Here's how the part is built. I have some questions about the finished solid (model axes, mm). A direction names the side the tool comes from. Round coordinates to 2 decimals unless told otherwise and drop trailing zeros. Write each loop counter-clockwise with the first axis right and the second up, starting at its lowest first coordinate (ties: lowest second). Pieces come first, ordered by that corner, then holes. Notation, with made-up numbers: M 61,-28.75 L 78,-28.75 A14 ccw 78,-2.75 Z; hole C 29,9.25 d2. An arc over 180 degrees is marked long. Write item = value, one per line. Start each with the question number.
(1) On a 3-axis mill with a long thin cutter (end or side, diameter ignored), from which of +Z, -Z, +X, -X, +Y, -Y can I reach the whole of each face in a straight line? I mean faces 1 (the flat face through (0, 25, 0)), 2 (the flat face through (-21.5, 14, -2)), 3 (the flat face through (18, 33, -21.75)), 4 (the cylindrical face through (-14.93, 4.52, 10.5)). Say none if no direction works.
(2) I want a section at C-C (y = 48). List the corners of the cut face in (x, z) for me, and give its area (3 significant figures).
(3) Will these pins go through, and if not, where does the flat tip stop? pin 1 Ø3 at (x, y) = (-16, 33.5) entering from +Z; pin 2 Ø6 at (x, z) = (3.5, -11.5) entering from +Y; pin 3 Ø1.4 at (x, z) = (-1.5, -29) entering from +Y; pin 4 Ø8 at (x, z) = (-12.5, -7) entering from -Y.
(4) I want a section at B-B (x = 0). List the corners of the cut face in (y, z) for me, and give its area (3 significant figures).
(5) I need wall thicknesses on line 1 along Z through (x, y) = (-15, 4.85); line 2 along Y through (x, z) = (-6.5, 17.5); line 3 along Z through (x, y) = (-11, 15). Which ranges of each line are inside material? Lowest first, please.
(6) If we mould it in two halves opening along Y, with no side actions, what happens to faces 5 (the conical face through (-15.159, 6.745, 12.207)), 6 (the flat face through (17.24, 1.48, 10.68)), 7 (the cylindrical face through (-15.268, 29.367, -20.614))? For each: released by +Y, released by -Y, zero draft, split by the parting line, or undercut.
(7) I want a section at D-D (y = 11.5). List the corners of the cut face in (x, z) for me.
(8) I want a section at A-A (z = 17.5). List the corners of the cut face in (x, y) for me, and give its area (3 significant figures).
```python
from build123d import *

# Parameters (mm, degrees)
SKETCH9_W                 = 43
SKETCH9_H                 = 27
BOSS_EXTRUDE1_DEPTH       = 32.5
CUT_EXTRUDE1_DEPTH        = 61.284741021
CUT_EXTRUDE1_DEPTH_BACK   = 61.284741021
SKETCH10_R                = 6
CUT_EXTRUDE2_DEPTH        = 3
CUT_EXTRUDE4_DEPTH        = 61.284741021
CUT_EXTRUDE4_DEPTH_BACK   = 61.284741021
SKETCH14_W                = 30
SKETCH14_H                = 2
SKETCH15_W                = 43
SKETCH15_H                = 6
BOSS_EXTRUDE2_DEPTH       = 43
F_3_0MM_DOWEL_HOLE1_D     = 3
F_3_0MM_DOWEL_HOLE1_DEPTH = 6
F_3_0MM_DOWEL_HOLE1_TIP   = 0.901290929
FILLET2_R                 = 10
SKETCH20_R                = 11
CUT_EXTRUDE5_DEPTH        = 2
CUT_EXTRUDE6_DEPTH        = 95.827804467
CUT_EXTRUDE6_DEPTH_BACK   = 95.827804467
SKETCH21_R                = 5
SKETCH21_R_2              = 1.5
SKETCH23_R                = 3
CUT_EXTRUDE7_DEPTH        = 6


with BuildPart() as part:
    # Sketch9 → Boss-Extrude1 (new, symmetric)
    with BuildSketch(Plane.XY):
        with Locations((0, 13.5)):
            Rectangle(SKETCH9_W, SKETCH9_H)
    extrude(amount=BOSS_EXTRUDE1_DEPTH, both=True)

    # Sketch10 → Cut-Extrude1 (cut, two sides: drawn at the far end of the back side and taken through both)
    with BuildSketch(Plane(origin=(21.5, 0, 0), x_dir=(0, 0, -1), z_dir=(1, 0, 0)).offset(-CUT_EXTRUDE1_DEPTH_BACK)):
        with Locations((-17.5, 15)):
            Circle(SKETCH10_R)
        with Locations(Location((17.5, 15, 0), (0, 0, 270))):
            Circle(SKETCH10_R)
    extrude(amount=CUT_EXTRUDE1_DEPTH + CUT_EXTRUDE1_DEPTH_BACK, mode=Mode.SUBTRACT)

    # Sketch11 → Cut-Extrude2 (cut)
    with BuildSketch(Plane.XZ):
        Polygon((12, -12), (13.5, -9.401923789), (16.5, -9.401923789), (18, -12), (16.5, -14.598076211), (13.5, -14.598076211), align=None)
        Polygon((13.5, 9.401923789), (16.5, 9.401923789), (18, 12), (16.5, 14.598076211), (13.5, 14.598076211), (12, 12), align=None)
        Polygon((-13.5, -9.401923789), (-16.5, -9.401923789), (-18, -12), (-16.5, -14.598076211), (-13.5, -14.598076211), (-12, -12), align=None)
        Polygon((-12, 12), (-13.5, 9.401923789), (-16.5, 9.401923789), (-18, 12), (-16.5, 14.598076211), (-13.5, 14.598076211), align=None)
    extrude(amount=-CUT_EXTRUDE2_DEPTH, mode=Mode.SUBTRACT)

    # Sketch14 → Cut-Extrude4 (cut, two sides: drawn at the far end of the back side and taken through both)
    with BuildSketch(Plane(origin=(21.5, 0, 0), x_dir=(0, 0, -1), z_dir=(1, 0, 0)).offset(-CUT_EXTRUDE4_DEPTH_BACK)):
        with Locations((0, 26)):
            Rectangle(SKETCH14_W, SKETCH14_H)
    extrude(amount=CUT_EXTRUDE4_DEPTH + CUT_EXTRUDE4_DEPTH_BACK, mode=Mode.SUBTRACT)

    # Sketch15 → Boss-Extrude2 (add)
    with BuildSketch(Plane(origin=(0, 27, 0), x_dir=(1, 0, 0), z_dir=(0, 1, 0))):
        with Locations((0, 24.75)):
            Rectangle(SKETCH15_W, SKETCH15_H)
    extrude(amount=BOSS_EXTRUDE2_DEPTH)

    # Ø3.0mm Dowel Hole1
    with Locations(Plane(origin=(15, 0, 12), x_dir=(0, 0, -1), z_dir=(0, -1, 0))):
        with Locations((0, 0), (0, -30), (24, -30), (24, 0)):
            Hole(F_3_0MM_DOWEL_HOLE1_D / 2, depth=F_3_0MM_DOWEL_HOLE1_DEPTH)
            with Locations((0, 0, -(F_3_0MM_DOWEL_HOLE1_DEPTH + F_3_0MM_DOWEL_HOLE1_TIP / 2))):  # 118° drill point
                Cone(0, F_3_0MM_DOWEL_HOLE1_D / 2, F_3_0MM_DOWEL_HOLE1_TIP, mode=Mode.SUBTRACT)

    # Fillet2
    # the kernel refuses this fillet: 10 mm, written as the material it adds along each edge
    with BuildSketch(Plane(origin=(21.5, 27, -21.75), x_dir=(0, 0, 1), z_dir=(-1, 0, 0))) as fillet2_piece_1:
        with BuildLine():
            CenterArc((10, 9.45714016), FILLET2_R, 180, 71.034425011)
            Line((0, 9.45714016), (-0.2, 9.45714016))
            Line((-0.2, 9.45714016), (-0.2, 0))
            Line((-0.2, 0), (0, -0.2))
            ThreePointArc((0, -0.2), (3.375, -0.2), (6.685, -0.189142803))
            Line((6.685, -0.189142803), (6.75, 0))
        make_face()
    extrude(amount=43)

    # Sketch20 → Cut-Extrude5 (cut)
    with BuildSketch(Plane(origin=(0, 0, -27.75), x_dir=(-1, 0, 0), z_dir=(0, 0, -1))):
        with Locations((0, 48)):
            Circle(SKETCH20_R)
    extrude(amount=-CUT_EXTRUDE5_DEPTH, mode=Mode.SUBTRACT)

    # Sketch21 → Cut-Extrude6 (cut, two sides: drawn at the far end of the back side and taken through both)
    with BuildSketch(Plane(origin=(0, 0, -27.75), x_dir=(-1, 0, 0), z_dir=(0, 0, -1)).offset(-CUT_EXTRUDE6_DEPTH_BACK)):
        with Locations((0, 48)):
            Circle(SKETCH21_R)
        with Locations((-16.341750707, 64.341750707)):
            Circle(SKETCH21_R_2)
        with Locations((15.658249293, 64.341750707)):
            Circle(SKETCH21_R_2)
        with Locations((15.658249293, 32.341750707)):
            Circle(SKETCH21_R_2)
        with Locations((-16.341750707, 32.341750707)):
            Circle(SKETCH21_R_2)
    extrude(amount=CUT_EXTRUDE6_DEPTH + CUT_EXTRUDE6_DEPTH_BACK, mode=Mode.SUBTRACT)

    # Sketch23 → Cut-Extrude7 (cut)
    with BuildSketch(Plane.XY.offset(-21.75)):
        with Locations(Location((-15.658249293, 32.341750707, 0), (0, 0, 180))):
            Circle(SKETCH23_R)
        with Locations(Location((16.341750707, 32.341750707, 0), (0, 0, 180))):
            Circle(SKETCH23_R)
    extrude(amount=CUT_EXTRUDE7_DEPTH, mode=Mode.SUBTRACT)


solid = part.part
```
Returned:
q1.face_1 = +X, -X, +Y
q1.face_2 = +Z, -Z, -X, +Y, -Y
q1.face_3 = +Z
q1.face_4 = -Y
q2.outline = M -21.5,-27.75 L -11,-27.75 L -11,-25.75 L -5,-25.75 L -5,-21.75 L -21.5,-21.75 Z; M 5,-25.75 L 11,-25.75 L 11,-27.75 L 21.5,-27.75 L 21.5,-21.75 L 5,-21.75 Z
q2.area = 174 mm²
q3.pin_1 = -21.75
q3.pin_2 = 25
q3.pin_3 = 27
q3.pin_4 = 0
q4.outline = M 0,-32.5 L 27,-32.5 L 27,-27.75 L 37,-27.75 L 37,-25.75 L 43,-25.75 L 43,-21.75 L 36.46,-21.75 A10 cw 27,-15 L 25,-15 L 25,15 L 27,15 L 27,32.5 L 0,32.5 Z; M 53,-25.75 L 59,-25.75 L 59,-27.75 L 70,-27.75 L 70,-21.75 L 53,-21.75 Z; hole C 15,-17.5 d12; hole C 15,17.5 d12
q4.area = 1,660 mm²
q5.line_1 = -32.5 to -13.5, -10.5 to 10.5, 13.5 to 32.5
q5.line_2 = 0 to 9, 21 to 27
q5.line_3 = -32.5 to -23.5, -11.5 to 11.5, 23.5 to 32.5
q6.face_5 = released by -Y
q6.face_6 = zero draft
q6.face_7 = undercut
q7.outline = M -21.5,-32.5 L 21.5,-32.5 L 21.5,-22.37 L -21.5,-22.37 Z; M -21.5,-12.63 L 21.5,-12.63 L 21.5,12.63 L -21.5,12.63 Z; M -21.5,22.37 L 21.5,22.37 L 21.5,32.5 L -21.5,32.5 Z
q8.outline = M -21.5,0 L 21.5,0 L 21.5,9 L -21.5,9 Z; M -21.5,21 L 21.5,21 L 21.5,27 L -21.5,27 Z
q8.area = 645 mm²
